```python
from build123d import *

# Parameters (mm, degrees)
PAD_DEPTH    = 5
SKETCH001_R  = 3
HOLE_DEPTH   = 5.001
POCKET_DEPTH = 5.001
FILLET_R     = 2


with BuildPart() as part:
    # Sketch → Pad (new body)
    with BuildSketch(Plane.XY):
        with BuildLine():
            Line((0, 0), (120, 0))
            Line((120, 0), (120, 30))
            Line((120, 30), (64, 30))
            ThreePointArc((40, 54), (47.029437, 37.029437), (64, 30))
            ThreePointArc((120, 134), (63.431458, 110.568542), (40, 54))
            ThreePointArc((120, 134), (140, 154), (120, 174))
            ThreePointArc((120, 174), (35.147186, 138.852814), (0, 54))
            Line((0, 0), (0, 54))
        make_face()
    extrude(amount=PAD_DEPTH)

    # Sketch001 (on Face10 of Pad) → Hole (cut, through all)
    with BuildSketch(Plane.XY.offset(5)):
        with Locations((15, 15)):
            Circle(SKETCH001_R)
        with Locations((100, 15)):
            Circle(SKETCH001_R)
    extrude(amount=-HOLE_DEPTH, mode=Mode.SUBTRACT)

    # Sketch002 (on Face5 of Hole) → Pocket (cut, through all)
    with BuildSketch(Plane.XY.offset(5)):
        with BuildLine():
            ThreePointArc((120, 157), (47.168002, 126.831998), (17, 54))
            ThreePointArc((17, 54), (20, 51), (23, 54))
            ThreePointArc((120, 151), (51.410642, 122.589358), (23, 54))
            ThreePointArc((120, 151), (123, 154), (120, 157))
        make_face()
    extrude(amount=-POCKET_DEPTH, mode=Mode.SUBTRACT)

    # Fillet
    fillet_edges = [part.edges().sort_by_distance(p)[0] for p in [
        (92, 30, 5),
        (92, 30, 0),
        (47.029437, 37.029437, 5),
        (63.431458, 110.568542, 5),
        (140, 154, 5),
        (35.147186, 138.852814, 5),
        (0, 27, 5),
        (47.029437, 37.029437, 0),
        (63.431458, 110.568542, 0),
        (140, 154, 0),
        (35.147186, 138.852814, 0),
        (0, 27, 0),
        (120, 15, 0),
        (120, 15, 5),
    ]]
    fillet(fillet_edges, radius=FILLET_R)


solid = part.part
```
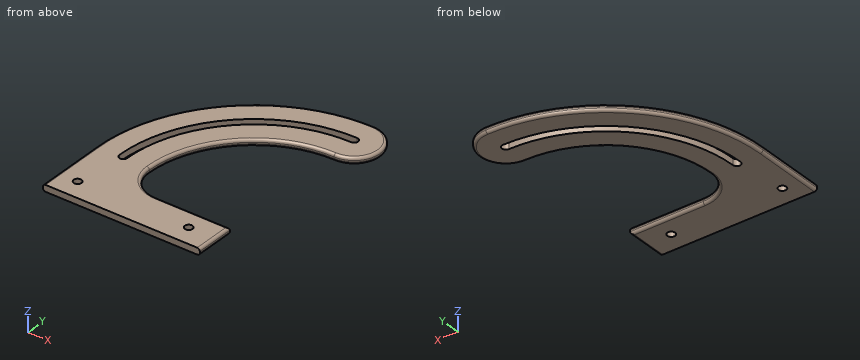
Design review of the part built by this model. Coordinates are the model's own, in mm. Coordinates: 2 decimals unless noted, no trailing zeros. Order: outer loops, then holes, each group sorted by start corner. A loop starts at its lowest first (then second) coordinate and runs counter-clockwise, first axis right, second up. Notation, with made-up numbers: (50, 83) - (73, 83) arc R29 ccw to (73, 115) - close; hole circle Ø5 at (-18, 11.25). An arc over 180 degrees is marked (long way). Answer in a Markdown table with one row per item.
(1) Wall thickness on line 1 along Y through (x, z) = (94, 0.7); line 2 along Y through (x, z) = (100, 2.7); line 3 along Y through (x, z) = (93.5, 4): over which ranges is each line inside the solid? List them lowest first. Write a range as from..to.
Checked values:
| item | result |
|---|---|
| line 1 | 0..29.52, 130.16..147.45, 153.66..170.66 |
| line 2 | 0..12, 18..30, 131.46..148.92, 155.04..172.32 |
| line 3 | 0..29.73, 129.77..147.31, 153.53..170.76 |
(2) Consider section B-B on z = 4.1. State the section outline as (x, y) points, plus the area to 3 significant figures.
Checked values:
| item | result |
|---|---|
| outline | (0.33, 0) - (119.67, 0) - (119.67, 29.67) - (64, 29.67) arc R24.33 cw to (39.67, 54) arc R80.33 cw to (120, 134.33) arc R19.67 ccw to (120, 173.67) arc R119.67 ccw to (0.33, 54) - close; hole circle Ø6 at (15, 15); hole (17, 54) arc R3 ccw to (23, 54) arc R97 cw to (120, 151) arc R3 ccw to (120, 157) arc R103 ccw to start; hole circle Ø6 at (100, 15) |
| area | 10,400 mm^2 |
(3) Clearance check with flat-ended pins moving along their axes: pin 1 (1.1 mm diameter, centred on y = 11.5, z = 2.5, fed in from +X); pin 2 (4 mm diameter, centred on x = 71.5, y = 22.5, fed in from -Z); pin 3 (3.5 mm diameter, centred on x = 100, y = 15, fed in from +Z); pin 4 (1.1 mm diameter, centred on x = 83.5, z = 2.5, fed in from +Y). State where each tip first meets the part, or that it passes through.
Checked values:
| item | result |
|---|---|
| pin 1 | x = 120 |
| pin 2 | z = 0 |
| pin 3 | through |
| pin 4 | y = 168.49 |
(4) Consider section C-C on x = 50. Give the number of separate pieces and of enclosed holes in the cut face, plus the area to 3 significant figures.
Checked values:
| item | result |
|---|---|
| separate pieces | 3 |
| enclosed holes | 0 |
| area | 416 mm^2 |
(5) Consider section A-A on y = 15. State the section outline as (x, z) points, plus the area to 3 significant figures.
Checked values:
| item | result |
|---|---|
| outline | (0, 2) arc R2 ccw to (2, 0) - (12, 0) - (12, 5) - (2, 5) arc R2 ccw to (0, 3) - close; (18, 0) - (97, 0) - (97, 5) - (18, 5) - close; (103, 0) - (118, 0) arc R2 ccw to (120, 2) - (120, 3) arc R2 ccw to (118, 5) - (103, 5) - close |
| area | 537 mm^2 |
